Design review of the part built by this model. Coordinates are the model's own, in mm. Round coordinates to 2 decimals unless told otherwise and drop trailing zeros. Order: outer loops, then holes, each group sorted by start corner. A loop starts at its lowest first (then second) coordinate and runs counter-clockwise, first axis right, second up. Notation, with made-up numbers: (71.25, -28.75) - (77.25, -28.75) arc R21 cw to (77.25, 3.25) - close; hole circle Ø11 at (24.5, 6.25). An arc over 180 degrees is marked (long way). Answer as a JSON object with one key per item and string values. Group by question number.
from build123d import *

# Parameters (mm, degrees)
CROQUIS1_R              = 47.5
SALIENTE_EXTRUIR1_DEPTH = 3
CROQUIS3_R              = 2
CROQUIS3_W              = 40
CROQUIS3_H              = 20
CORTAR_EXTRUIR1_DEPTH   = 4
CROQUIS4_R              = 1.5
CORTAR_EXTRUIR2_DEPTH   = 4


with BuildPart() as part:
    # Croquis1 → Saliente-Extruir1 (new body)
    with BuildSketch(Plane.XY):
        Circle(CROQUIS1_R)
    extrude(amount=SALIENTE_EXTRUIR1_DEPTH)

    # Croquis3 → Cortar-Extruir1 (cut, through all)
    with BuildSketch(Plane.XY.offset(3)):
        with Locations((35, -5)):
            Circle(CROQUIS3_R)
        with Locations((35, 5)):
            Circle(CROQUIS3_R)
        with Locations((-15.5, -5)):
            Circle(CROQUIS3_R)
        with Locations((-15.5, 5)):
            Circle(CROQUIS3_R)
        with Locations((9.75, 0)):
            Rectangle(CROQUIS3_W, CROQUIS3_H)
    extrude(amount=-CORTAR_EXTRUIR1_DEPTH, mode=Mode.SUBTRACT)

    # Croquis4 → Cortar-Extruir2 (cut, through all)
    with BuildSketch(Plane.XY.offset(3)):
        with Locations((-42.5, 0)):
            Circle(CROQUIS4_R)
        with Locations((-13.133222261, 40.419901943)):
            Circle(CROQUIS4_R)
        with Locations((34.383222261, 24.980873222)):
            Circle(CROQUIS4_R)
        with Locations((34.383222261, -24.980873222)):
            Circle(CROQUIS4_R)
        with Locations((-13.133222261, -40.419901943)):
            Circle(CROQUIS4_R)
    extrude(amount=-CORTAR_EXTRUIR2_DEPTH, mode=Mode.SUBTRACT)


solid = part.part
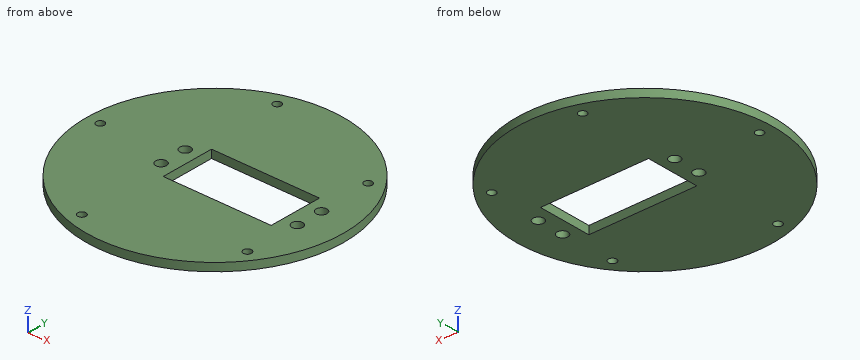
1. To check wall thickness, follow line 1 (Y direction, x = 0.5, z = 2.6); line 2 (X direction, y = 6.5, z = 2.2); line 3 (Y direction, x = -14, z = 2.65). State the ranges of each line that lie inside material, in increasing order. Write a range as from..to.
2. Take a section at C-C, the plane z = 1.4. Count the separate pieces of the cut face and the enclosed holes in it, then the cut area to 3 significant figures.
3. Take a section at B-B, the plane x = -42.5. Give the boundary of the cut face in (y, z), then the cut area to 3 significant figures.
4. Take a section at A-A, the plane y = 0. Give the boundary of the cut face in (x, z).
5. Clearance check with flat-ended pins moving along their axes: P1, Ø5, axis at x = 34.38, y = -24.98, coming from the +Z side; P2, Ø1.5, axis at y = 19, z = 1, coming from the +X side; P3, Ø1.5, axis at x = 15.5, z = 2, coming from the +Y side; P4, Ø2.5, axis at x = -13.13, y = -40.42, coming from the -Z side. State where each tip first meets the part, or that it passes through.
6. Take a section at D-D, the plane x = 13.5. Give the boundary of the cut face in (y, z).
Response values:
{
 "1": {"line 1": "-47.5..-10, 10..47.5", "line 2": "-47.05..-16.82, -14.18..-10.25, 29.75..33.68, 36.32..47.05", "line 3": "-45.39..-41.64, -39.2..-6.32, -3.68..3.68, 6.32..39.2, 41.64..45.39"},
 "2": {"separate pieces": "1", "enclosed holes": "10", "area": "6,200 mm2"},
 "3": {"outline": "(-21.21, 0) - (-1.5, 0) - (-1.5, 3) - (-21.21, 3) - close; (1.5, 0) - (21.21, 0) - (21.21, 3) - (1.5, 3) - close", "area": "118 mm2"},
 "4": {"outline": "(-47.5, 0) - (-44, 0) - (-44, 3) - (-47.5, 3) - close; (-41, 0) - (-10.25, 0) - (-10.25, 3) - (-41, 3) - close; (29.75, 0) - (47.5, 0) - (47.5, 3) - (29.75, 3) - close"},
 "5": {"P1": "z = 3", "P2": "x = 43.85", "P3": "y = 45.15", "P4": "through"},
 "6": {"outline": "(-45.54, 0) - (-10, 0) - (-10, 3) - (-45.54, 3) - close; (10, 0) - (45.54, 0) - (45.54, 3) - (10, 3) - close"}
}
